Model file for the job. Use its own axes, mm. Round coordinates to 2 decimals unless told otherwise and drop trailing zeros. Order: outer loops, then holes, each group sorted by start corner. A loop starts at its lowest first (then second) coordinate and runs counter-clockwise, first axis right, second up. Notation, with made-up numbers: (-35.75, -21.75) -> (-18.75, -21.75) arc R27 cw to (-18.75, 4.25) -> close; hole circle Ø3 at (56.5, -35). An arc over 180 degrees is marked (long way). Put each result on its own line as item: value. Start each with the question number.
Q1. Probe L1, parallel to X at y = 2.5, z = 0.4; L2, parallel to X at y = -6.5, z = 1.15; L3, parallel to Y at x = 37, z = 0.6. List the from-to ranges inside material, lowest first.
Q2. Cut at A-A, the plane x = 8. List the corners of the cut face in (y, z).
Q3. Pull direction Y, two halves, no side cores. Call faces 1 (the face through (39.93, 0.04, 1)), 2 (the face through (26, 0, 0)), 3 (the face through (29, -13.5, 1)), 4 (the face through (0.854, -9.641, 1.002)): released by +Y, released by -Y, zero draft, split by the parting line, or undercut.
Q4. Cut at C-C, the plane x = 52.5. List the corners of the cut face in (y, z), and give its area (3 significant figures).
Q5. Cut at B-B, the plane z = 0.65. State how many separate pieces and enclosed holes the cut face has, and give its area (3 significant figures).
Q6. Flat gauge pins, fed straight in: P1, Ø1, axis at x = 52, z = 0.5, coming from the +Y side; P2, Ø1, axis at x = 29, z = 0.5, coming from the +Y side. Where does each tip first touch, or does it go through?
from build123d import *

# Parameters (mm, degrees)
SKETCH2_R           = 1.85
SKETCH2_R_2         = 1.35255
SKETCH2_R_3         = 4
SKETCH2_R_4         = 1.5875
BOSS_EXTRUDE1_DEPTH = 2.032


with BuildPart() as part:
    # Sketch2 → Boss-Extrude1 (new body)
    with BuildSketch(Plane.XY):
        with BuildLine():
            Line((45.396235039, 13.510064828), (45.386170211, 13.5))
            Line((45.386170211, 13.5), (0, 13.5))
            ThreePointArc((0, 13.5), (-13.5, 0), (0, -13.5))
            Line((0, -13.5), (59.39836352, -13.5))
            Line((59.39836352, -13.5), (65.902331694, -6.996031827))
            Line((65.902331694, -6.996031827), (45.396235039, 13.510064828))
        make_face()
        with Locations((8, 0)):
            Circle(SKETCH2_R, mode=Mode.SUBTRACT)
        with Locations((55.883335711, -7.214527822)):
            Circle(SKETCH2_R_2, mode=Mode.SUBTRACT)
        with Locations((45.107028366, 3.561779523)):
            Circle(SKETCH2_R_2, mode=Mode.SUBTRACT)
        Circle(SKETCH2_R_3, mode=Mode.SUBTRACT)
        with Locations((0, -8)):
            Circle(SKETCH2_R, mode=Mode.SUBTRACT)
        with Locations((-8, 0)):
            Circle(SKETCH2_R, mode=Mode.SUBTRACT)
        with Locations((0, 8)):
            Circle(SKETCH2_R, mode=Mode.SUBTRACT)
        with Locations((41.514925917, -0.030322925)):
            Circle(SKETCH2_R_4, mode=Mode.SUBTRACT)
        with Locations((52.291233263, -10.80663027)):
            Circle(SKETCH2_R_4, mode=Mode.SUBTRACT)
    extrude(amount=BOSS_EXTRUDE1_DEPTH)


solid = part.part
Ans:
1. L1: x = -13.27 to -3.12, 3.12 to 44.27, 45.94 to 56.41
1. L2: x = -11.83 to -1.08, 1.08 to 54.73, 57.03 to 65.41
1. L3: y = -13.5 to 13.5
2. outline: (-13.5, 0) -> (-1.85, 0) -> (-1.85, 2.03) -> (-13.5, 2.03) -> close; (1.85, 0) -> (13.5, 0) -> (13.5, 2.03) -> (1.85, 2.03) -> close
3. face 1: undercut
3. face 2: zero draft
3. face 3: released by -Y
3. face 4: undercut
4. outline: (-13.5, 0) -> (-12.38, 0) -> (-12.38, 2.03) -> (-13.5, 2.03) -> close; (-9.23, 0) -> (6.41, 0) -> (6.41, 2.03) -> (-9.23, 2.03) -> close
4. area: 34.1 mm^2
5. separate pieces: 1
5. enclosed holes: 9
5. area: 1,710 mm^2
6. P1: stops at y = 7.41
6. P2: stops at y = 13.5
